Part print with two shaded views. Sizes in mm from the minimum x, y, z corner. Round coordinates to 2 decimals unless told otherwise and drop trailing zeros. Order: outer loops, then holes, each group sorted by start corner. A loop starts at its lowest first (then second) coordinate and runs counter-clockwise, first axis right, second up. Notation, with made-up numbers: M 82,4 L 102,4 A20 ccw 102,41 Z; hole C -38.5,28.5 d11. An arc over 180 degrees is marked long. Answer as a JSON object with one key per item and string values.
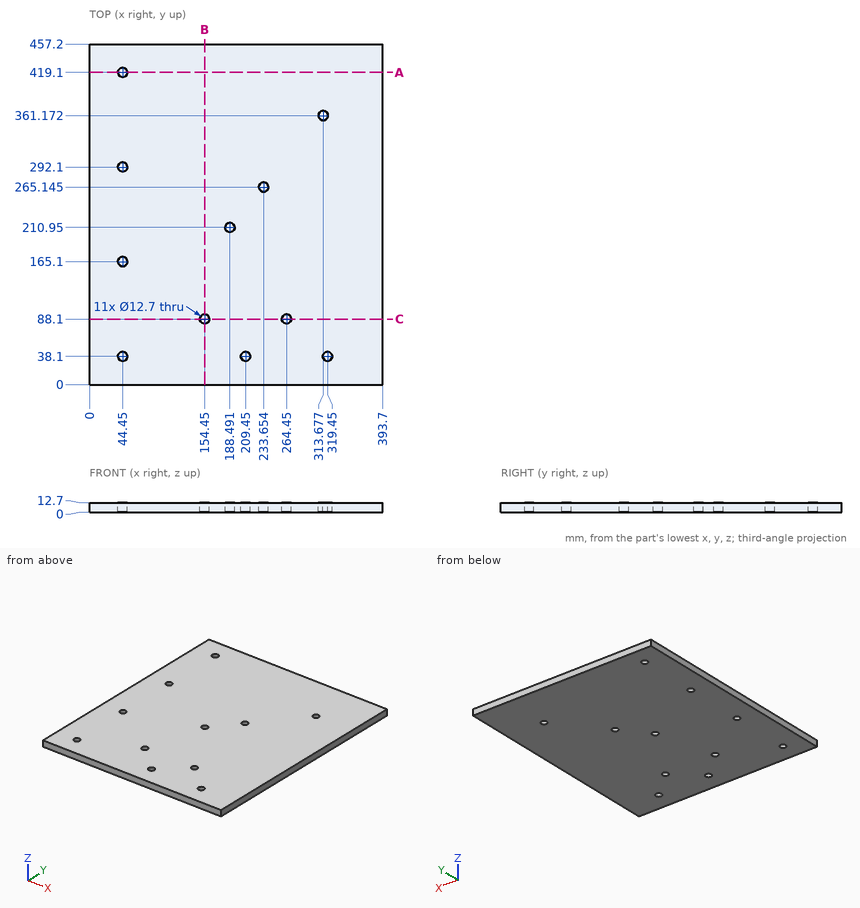
Item 1: Saw through at B-B on x = 154.45. List the corners of the cut face in (y, z).
Worked answers:
{"outline": "M 0,0 L 81.75,0 L 81.75,12.7 L 0,12.7 Z; M 94.45,0 L 457.2,0 L 457.2,12.7 L 94.45,12.7 Z"}
Item 2: Wall check: line 1 along X through (y, z) = (88.1, 7); line 2 along Y through (x, z) = (44.45, 3.25); line 3 along X through (y, z) = (38.1, 8.75). Give the ranges that are in metal, low to high. Write a range as [from, to].
Worked answers:
{"line 1": "x = [0, 148.1], [160.8, 258.1], [270.8, 393.7]", "line 2": "y = [0, 31.75], [44.45, 158.75], [171.45, 285.75], [298.45, 412.75], [425.45, 457.2]", "line 3": "x = [0, 38.1], [50.8, 203.1], [215.8, 313.1], [325.8, 393.7]"}
Item 3: Saw through at C-C on y = 88.1. List the corners of the cut face in (x, z), and give its area (3 significant figures).
Worked answers:
{"outline": "M 0,0 L 148.1,0 L 148.1,12.7 L 0,12.7 Z; M 160.8,0 L 258.1,0 L 258.1,12.7 L 160.8,12.7 Z; M 270.8,0 L 393.7,0 L 393.7,12.7 L 270.8,12.7 Z", "area": "4,680 mm2"}
Item 4: Drop a flat-ended pin along its axis: pin 1 Ø10 at (x, y) = (44.45, 165.1) entering from -Z. Give the stop position or say it passes through.
Worked answers:
{"pin 1": "passes through"}
Item 5: Saw through at A-A on y = 419.1. List the corners of the cut face in (x, z), and give its area (3 significant figures).
Worked answers:
{"outline": "M 0,0 L 38.1,0 L 38.1,12.7 L 0,12.7 Z; M 50.8,0 L 393.7,0 L 393.7,12.7 L 50.8,12.7 Z", "area": "4,840 mm2"}
